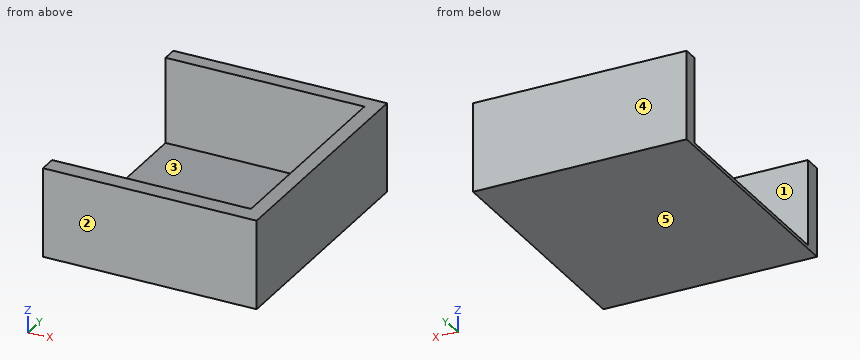
```python
from build123d import *

# Parameters (mm, degrees)
F0_W     = 102.33476
F0_H     = 110.469941
F1_DEPTH = 39.37
F2_W     = 88.028256
F2_H     = 96.191108
F3_DEPTH = 37.846
F4_W     = 28.833367
F4_H     = 140.770766
F5_DEPTH = 58.166


with BuildPart() as f1:
    # F0 (on Top) → F1 (new body)
    with BuildSketch(Plane.XY):
        with Locations((-1.762386, 3.01904)):
            Rectangle(F0_W, F0_H)
    extrude(amount=-F1_DEPTH)

    # F2 (on face) → F3 (cut)
    with BuildSketch(Plane.XY):
        with Locations((-1.146434, 3.571052)):
            Rectangle(F2_W, F2_H)
    extrude(amount=-F3_DEPTH, mode=Mode.SUBTRACT)

    # F4 (on Top) → F5 (cut)
    with BuildSketch(Plane.XY):
        with Locations((-59.548001, 17.85939)):
            Rectangle(F4_W, F4_H)
    extrude(amount=-F5_DEPTH, mode=Mode.SUBTRACT)


solid = f1.part
```
Model file for the job. Use its own axes, mm. Face numbers are marked on the shaded views. A direction names the side the tool comes from. Coordinates: 2 decimals unless noted, no trailing zeros. Loops run counter-clockwise (first coordinate to the right, second up) from the corner with the lowest first, then second, coordinate; pieces in that order, holes last. Notation, with made-up numbers: (32.25, 89.25) - (38.25, 89.25) arc R27 cw to (38.25, 117.25) - close; hole circle Ø9 at (46.5, 74). An arc over 180 degrees is marked (long way). Answer as a JSON object with one key per item and string values. Group by question number.
(1) Two-plate mould, pull along Y, no slides. Class the marked faces 3, 4 and 5: released by +Y, released by -Y, zero draft, split by the parting line, or undercut.
(2) Probe line 1 along Y through (x, z) = (4.5, -7); line 2 along Z through (x, y) = (-3, 30); line 3 along X through (y, z) = (47.5, -14.5) (3 decimals). List the from-to ranges inside material, lowest first.
(3) Tool access for the marked faces 1 and 2: list every direction of +Z, -Z, +X, -X, +Y, -Y with a clear straight run to the whole face (end or side of a thin tool).
(4) Cut at C-C (y = 22). Give the cut face in (x, z) (3 decimals), then the cut area to 3 significant figures.
(5) Cut at B-B (x = 13). Give the cut face in (y, z), then the cut area to 3 significant figures.
(6) Flat gauge pin, fed straight in: pin 1 (5 mm diameter, centred on y = 13, z = -29.5, fed in from -X). Where does the tip first touch, or does it go through?
(7) Cut at A-A (z = -22). Give the cut face in (x, y) (1 decimal).
Geometry says:
{
 "1": {"face 3": "undercut", "face 4": "released by +Y", "face 5": "zero draft"},
 "2": {"line 1": "y = -52.22 to -44.52, 51.67 to 58.25", "line 2": "z = -39.37 to -37.85", "line 3": "x = 42.868 to 49.405"},
 "3": {"face 1": "+Z, -X", "face 2": "+Z, -Z, +X, -X, -Y"},
 "4": {"outline": "(-45.131, -39.37) - (49.405, -39.37) - (49.405, 0) - (42.868, 0) - (42.868, -37.846) - (-45.131, -37.846) - close", "area": "391 mm^2"},
 "5": {"outline": "(-52.22, -39.37) - (58.25, -39.37) - (58.25, 0) - (51.67, 0) - (51.67, -37.85) - (-44.52, -37.85) - (-44.52, 0) - (-52.22, 0) - close", "area": "709 mm^2"},
 "6": {"pin 1": "stops at x = 42.87"},
 "7": {"outline": "(-45.1, -52.2) - (49.4, -52.2) - (49.4, 58.3) - (-45.1, 58.3) - (-45.1, 51.7) - (42.9, 51.7) - (42.9, -44.5) - (-45.1, -44.5) - close"}
}
